Check sheet for the modelled part. Datum: model origin and axes. Units: mm. A direction names the side the tool comes from. Coordinates: 2 decimals unless noted, no trailing zeros. Order: outer loops, then holes, each group sorted by start corner. A loop starts at its lowest first (then second) coordinate and runs counter-clockwise, first axis right, second up.
from build123d import *

# Parameters (mm, degrees)
SKETCH9_W           = 95
SKETCH9_H           = 55
BOSS_EXTRUDE1_DEPTH = 90
CUT_EXTRUDE5_DEPTH  = 100
SKETCH12_W          = 60.486878253
SKETCH12_H          = 73.853608548
CUT_EXTRUDE7_DEPTH  = 80
SKETCH13_W          = 80
SKETCH13_H          = 25.917714192
CUT_EXTRUDE8_DEPTH  = 22.845479
FILLET1_R           = 20
SKETCH16_R          = 7.5
CUT_EXTRUDE9_DEPTH  = 30
SKETCH17_W          = 37
SKETCH17_H          = 20
CUT_EXTRUDE10_DEPTH = 30
SKETCH18_R          = 7.5
CUT_EXTRUDE11_DEPTH = 30


with BuildPart() as part:
    # Sketch9 → Boss-Extrude1 (new body)
    with BuildSketch(Plane(origin=(0, 0, 0), x_dir=(1, 0, 0), z_dir=(0, 1, 0))):
        with Locations((9.391117479, -20.408309456)):
            Rectangle(SKETCH9_W, SKETCH9_H)
    extrude(amount=-BOSS_EXTRUDE1_DEPTH)

    # Sketch10 → Cut-Extrude5 (cut)
    with BuildSketch(Plane(origin=(56.891117479, 0, 0), x_dir=(0, 0, -1), z_dir=(1, 0, 0))):
        with BuildLine():
            ThreePointArc((-6.717440326, -0.405285552), (1.502612431, -4.261054452), (7.091690544, -11.416362061))
            Line((7.091690544, -11.416362061), (7.091690544, 0))
            Line((7.091690544, 0), (-6.717440326, 0))
            Line((-6.717440326, 0), (-6.717440326, -0.405285552))
        make_face()
        with BuildLine():
            Line((-47.908309456, -77.945973927), (-29.335605617, -77.945973927))
            Line((-29.335605617, -77.945973927), (-29.335605617, -13.754463437))
            ThreePointArc((-29.335605617, -13.754463437), (-22.266542801, -3.810210472), (-10.675938318, 0))
            Line((-10.675938318, 0), (-47.908309456, 0))
            Line((-47.908309456, 0), (-47.908309456, -77.945973927))
        make_face()
    extrude(amount=-CUT_EXTRUDE5_DEPTH, mode=Mode.SUBTRACT)

    # Sketch12 → Cut-Extrude7 (cut)
    with BuildSketch(Plane.ZY.offset(38.108882521)):
        with Locations((7.902207673, -18.173690635)):
            Rectangle(SKETCH12_W, SKETCH12_H)
    extrude(amount=-CUT_EXTRUDE7_DEPTH, mode=Mode.SUBTRACT)

    # Sketch13 → Cut-Extrude8 (cut)
    with BuildSketch(Plane(origin=(0, -55.100494909, 0), x_dir=(1, 0, 0), z_dir=(0, 1, 0))):
        with Locations((1.891117479, -16.376748521)):
            Rectangle(SKETCH13_W, SKETCH13_H)
    extrude(amount=-CUT_EXTRUDE8_DEPTH, mode=Mode.SUBTRACT)

    # Fillet1
    fillet1_edges = [part.edges().sort_by_distance(p)[0] for p in [
        (41.891117479, -55.100494909, -1.836899559),
    ]]
    fillet(fillet1_edges, radius=FILLET1_R)

    # Sketch16 → Cut-Extrude9 (cut)
    with BuildSketch(Plane.XY.offset(3.417891425)):
        with Locations((-23.342301778, -66.523234418)):
            Circle(SKETCH16_R)
        with Locations((27.03315513, -66.523234418)):
            Circle(SKETCH16_R)
    extrude(amount=-CUT_EXTRUDE9_DEPTH, mode=Mode.SUBTRACT)

    # Sketch17 → Cut-Extrude10 (cut)
    with BuildSketch(Plane(origin=(0, -77.945973927, 0), x_dir=(1, 0, 0), z_dir=(0, 1, 0))):
        with Locations((1.421785082, -18.172095262)):
            Rectangle(SKETCH17_W, SKETCH17_H)
    extrude(amount=-CUT_EXTRUDE10_DEPTH, mode=Mode.SUBTRACT)

    # Sketch18 → Cut-Extrude11 (cut)
    with BuildSketch(Plane.ZY.offset(-41.891117479)):
        with Locations((11.481013295, -14.392127448)):
            Circle(SKETCH18_R)
    extrude(amount=-CUT_EXTRUDE11_DEPTH, mode=Mode.SUBTRACT)


solid = part.part
(1) Go/stop test with flat-tipped pins: P1, Ø13.5, axis at x = -23.34, y = -66.52, coming from the -Z side; P2, Ø13, axis at x = 2.5, y = -57, coming from the +Z side; P3, Ø2, axis at y = -21, z = 11.5, coming from the -X side; P4, Ø12, axis at x = -8.5, z = 3.5, coming from the +Y side. Record where each tip stops, or that it passes through.
Filled in:
P1: passes through
P2: stops at z = 3.42
P3: stops at x = 41.89
P4: stops at y = -55.1
(2) Cross-section at B-B (y = -10). Enter the section's corners in (x, z), and give its area (3 significant figures).
Filled in:
outline: (41.89, -6.37) - (56.89, -6.37) - (56.89, 5.4) - (41.89, 5.4) - close; (41.89, 17.56) - (56.89, 17.56) - (56.89, 27.73) - (41.89, 27.73) - close
area: 329 mm2
(3) Release check for a two-part mould opening along X. For faces 5 (the cylindrical face through (-24.319, -59.087, -1.763)), 6 (the flat face through (19, -68, -7.092)), 7 (the flat face through (41.891, -38, 15)) record: +X half, -X half, draft (parallel to the pull), parting line (faces both ways), or undercut.
Filled in:
face 5: undercut
face 6: draft
face 7: -X half
(4) Cross-section at C-C (z = 26). Enter the section's corners in (x, y), and give its area (3 significant figures).
Filled in:
outline: (-38.11, -90) - (-17.08, -90) - (-17.08, -77.95) - (-38.11, -77.95) - close; (19.92, -90) - (56.89, -90) - (56.89, -7.42) - (41.89, -7.42) - (41.89, -77.95) - (19.92, -77.95) - close
area: 1,760 mm2
(5) Cross-section at D-D (z = 12.5). Enter the section's corners in (x, y), and give its area (3 significant figures).
Filled in:
outline: (-38.11, -90) - (-17.08, -90) - (-17.08, -77.95) - (-38.11, -77.95) - close; (19.92, -90) - (56.89, -90) - (56.89, -21.82) - (41.89, -21.82) - (41.89, -77.95) - (19.92, -77.95) - close; (41.89, -6.96) - (56.89, -6.96) - (56.89, -0.09) - (41.89, -0.09) - close
area: 1,640 mm2
(6) Cross-section at A-A (x = -7.5). Enter the section's corners in (y, z).
Filled in:
outline: (-90, -7.09) - (-55.1, -7.09) - (-55.1, 3.42) - (-77.95, 3.42) - (-77.95, 8.17) - (-90, 8.17) - close; (-90, 28.17) - (-77.95, 28.17) - (-77.95, 47.91) - (-90, 47.91) - close
(7) Tool access check on faces 1 (the cylindrical face through (26.057, -59.087, -1.763)), 2 (the flat face through (-9, -55.1, -2)), 3 (the flat face through (1, -66, 3.418)), 4 (the flat face through (-17.078, -84, 18)). Record the directions out of +Z, -Z, +X, -X, +Y, -Y that give a thin tool (end or side, any length) a straight path to the whole face; none if there is none.
Filled in:
face 1: +Z, -Z
face 2: +Z, -Z, -X, +Y
face 3: +Z, -X, +Y
face 4: +Y, -Y
(8) Thickness scan on probe 1 along X at (y, z) = (-78, 26); probe 2 along X at (y, z) = (-72, 1); probe 3 along X at (y, z) = (-71, -0.5). Record the ranges inside material, lowest first.
Filled in:
probe 1: x = -38.11 to -17.08, 19.92 to 56.89
probe 2: x = -38.11 to -28.47, -18.22 to 21.91, 32.16 to 56.89
probe 3: x = -38.11 to -29.36, -17.32 to 21.02, 33.05 to 56.89
